from build123d import *

# Parameters (mm, degrees)
BOSS_EXTRUDE1_DEPTH            = 15
CUT_EXTRUDE1_DEPTH             = 5
CBORE_FOR_M3_SHCS1_D           = 3.4
CBORE_FOR_M3_SHCS1_CBORE_D     = 6.5
CBORE_FOR_M3_SHCS1_CBORE_DEPTH = 3
CRVPATTERN1_START              = -15
CRVPATTERN1_OUTLINE_R          = 1.7
CRVPATTERN1_DEPTH              = 30
CRVPATTERN1_START_2            = 12
CRVPATTERN1_2_OUTLINE_R        = 3.25
CRVPATTERN1_2_OUTLINE_R_2      = 1.7
CRVPATTERN1_2_DEPTH            = 3


# Read off the part's stored shape, not the designer's step: CrvPattern1
with BuildPart() as part:
    # Sketch1 → Boss-Extrude1 (new, symmetric)
    with BuildSketch(Plane.XY):
        with BuildLine():
            Line((-100.2, 0), (-100.2, -70))
            Line((-100.2, -70), (-120.2, -70))
            Line((-120.2, -70), (-120.2, 120))
            Line((-120.2, 120), (120.2, 120))
            Line((120.2, 120), (120.2, -70))
            Line((120.2, -70), (100.2, -70))
            Line((100.2, -70), (100.2, 0))
            ThreePointArc((100.2, 0), (0, 100.2), (-100.2, 0))
        make_face()
    extrude(amount=BOSS_EXTRUDE1_DEPTH, both=True)

    # Sketch2 → Cut-Extrude1 (cut, symmetric)
    with BuildSketch(Plane.XY):
        with BuildLine():
            Line((-110.2, -70), (-110.2, 0))
            ThreePointArc((-110.2, 0), (0, 110.2), (110.2, 0))
            Line((110.2, 0), (110.2, -70))
            Line((110.2, -70), (100.2, -70))
            Line((100.2, -70), (100.2, 0))
            ThreePointArc((100.2, 0), (0, 100.2), (-100.2, 0))
            Line((-100.2, 0), (-100.2, -70))
            Line((-100.2, -70), (-110.2, -70))
        make_face()
    extrude(amount=CUT_EXTRUDE1_DEPTH, both=True, mode=Mode.SUBTRACT)

    # CBORE for M3 SHCS1 (through all)
    with Locations(Plane.XY.offset(15)):
        with Locations((-105.2, -55)):
            CounterBoreHole(CBORE_FOR_M3_SHCS1_D / 2, CBORE_FOR_M3_SHCS1_CBORE_D / 2, CBORE_FOR_M3_SHCS1_CBORE_DEPTH)

    # CrvPattern1 outline → CrvPattern1 (cut)
    with BuildSketch(Plane.XY.offset(CRVPATTERN1_START)):
        with Locations((-103.59220022, 18.322010084)):
            Circle(CRVPATTERN1_OUTLINE_R)
        with Locations((-67.600164716, 80.605568855)):
            Circle(CRVPATTERN1_OUTLINE_R)
        with Locations((0, 105.2)):
            Circle(CRVPATTERN1_OUTLINE_R)
        with Locations((67.600164716, 80.605568855)):
            Circle(CRVPATTERN1_OUTLINE_R)
        with Locations((103.59220022, 18.322010084)):
            Circle(CRVPATTERN1_OUTLINE_R)
        with Locations((105.2, -55)):
            Circle(CRVPATTERN1_OUTLINE_R)
    extrude(amount=CRVPATTERN1_DEPTH, mode=Mode.SUBTRACT)

    # CrvPattern1 2 outline → CrvPattern1 2 (cut)
    # profile 1 of 6: a face of its own
    with BuildSketch(Plane.XY.offset(CRVPATTERN1_START_2)):
        with Locations((-103.59220022, 18.322010084)):
            Circle(CRVPATTERN1_2_OUTLINE_R)
        with Locations((-103.59220022, 18.322010084)):
            Circle(CRVPATTERN1_2_OUTLINE_R_2, mode=Mode.SUBTRACT)
    # profile 2 of 6: a face of its own
    with BuildSketch(Plane.XY.offset(CRVPATTERN1_START_2)):
        with Locations((-67.600164716, 80.605568855)):
            Circle(CRVPATTERN1_2_OUTLINE_R)
        with Locations((-67.600164716, 80.605568855)):
            Circle(CRVPATTERN1_2_OUTLINE_R_2, mode=Mode.SUBTRACT)
    # profile 3 of 6: a face of its own
    with BuildSketch(Plane.XY.offset(CRVPATTERN1_START_2)):
        with Locations((0, 105.2)):
            Circle(CRVPATTERN1_2_OUTLINE_R)
        with Locations((0, 105.2)):
            Circle(CRVPATTERN1_2_OUTLINE_R_2, mode=Mode.SUBTRACT)
    # profile 4 of 6: a face of its own
    with BuildSketch(Plane.XY.offset(CRVPATTERN1_START_2)):
        with Locations((67.600164716, 80.605568855)):
            Circle(CRVPATTERN1_2_OUTLINE_R)
        with Locations((67.600164716, 80.605568855)):
            Circle(CRVPATTERN1_2_OUTLINE_R_2, mode=Mode.SUBTRACT)
    # profile 5 of 6: a face of its own
    with BuildSketch(Plane.XY.offset(CRVPATTERN1_START_2)):
        with Locations((103.59220022, 18.322010084)):
            Circle(CRVPATTERN1_2_OUTLINE_R)
        with Locations((103.59220022, 18.322010084)):
            Circle(CRVPATTERN1_2_OUTLINE_R_2, mode=Mode.SUBTRACT)
    # profile 6 of 6: a face of its own
    with BuildSketch(Plane.XY.offset(CRVPATTERN1_START_2)):
        with Locations((105.2, -55)):
            Circle(CRVPATTERN1_2_OUTLINE_R)
        with Locations((105.2, -55)):
            Circle(CRVPATTERN1_2_OUTLINE_R_2, mode=Mode.SUBTRACT)
    extrude(amount=CRVPATTERN1_2_DEPTH, mode=Mode.SUBTRACT)


solid = part.part
Geometry check sheet. Reference: the model listing, model coordinates, mm. A direction names the side the tool comes from. Give positions to 0.01 mm unless a question says otherwise; leave off trailing zeros. Loops run counter-clockwise (first coordinate to the right, second up) from the corner with the lowest first, then second, coordinate; pieces in that order, holes last. Notation, with made-up numbers: (10.5, 86.25) -> (20.5, 86.25) arc R27 cw to (20.5, 107.25) -> close; hole circle Ø8 at (52, -17). An arc over 180 degrees is marked (long way). Answer in a Markdown table with one row per item. Add a question column.
1) Cross-section at B-B on z = 0.25. Record the boundary of the cut face in (x, y).
2) Set-up check for faces 4 (the face through (100.2, -35, 10)), 5 (the face through (1, 101, 5)), 6 (the face through (67.18, 83.83, 13.48)), 7 (the face through (113, -70, 0)): record each of +Z, -Z, +X, -X, +Y, -Y from which the full face is reachable in a straight line by a thin tool's end or side.
3) Gauge pin test, flat ends, axial feed: P1, Ø3, axis at x = 68, y = 81.5, coming from the +Z side; P2, Ø10, axis at x = 75.5, z = -3, coming from the -Y side. Record the tip position at first contact, or that the pin passes through.
4) Material ranges on probe 1 along Z at (x, y) = (-102.5, -56.5); probe 2 along X at (y, z) = (75.5, -6.75); probe 3 along X at (y, z) = (-30, 4.75), recorded low to high. Write a range as from..to.
5) Cross-section at C-C on x = -51. Record the boundary of the cut face in (y, z).
6) Draft check along Z on faces 1 (the face through (108.3, -54.02, 13.48)), 2 (the face through (1, 101, -5)), 3 (the face through (2, 111, 15)). Enter one of: pulls with the +Z half, pulls with the -Z half, needs draft (parallel to the pull), parting line crosses it, or undercut.
7) Cross-section at A-A on y = 56. Record the boundary of the cut face in (x, z).
Outcome:
| question | item | result |
|---|---|---|
| 1 | outline | (-120.2, -70) -> (-110.2, -70) -> (-110.2, 0) arc R110.2 cw to (110.2, 0) -> (110.2, -70) -> (120.2, -70) -> (120.2, 120) -> (-120.2, 120) -> close |
| 2 | face 4 | +Z, -Z, -Y |
| 2 | face 5 | -Y |
| 2 | face 6 | +Z |
| 2 | face 7 | +Z, -Z, +X, -X, -Y |
| 3 | P1 | stops at z = 12 |
| 3 | P2 | stops at y = 60.22 |
| 4 | probe 1 | z = -15..-5, 5..12 |
| 4 | probe 2 | x = -120.2..-65.88, 65.88..120.2 |
| 4 | probe 3 | x = -120.2..-110.2, 110.2..120.2 |
| 5 | outline | (86.25, -15) -> (120, -15) -> (120, 15) -> (86.25, 15) -> (86.25, 5) -> (97.69, 5) -> (97.69, -5) -> (86.25, -5) -> close |
| 6 | face 1 | needs draft |
| 6 | face 2 | undercut |
| 6 | face 3 | pulls with the +Z half |
| 7 | outline | (-120.2, -15) -> (-83.09, -15) -> (-83.09, -5) -> (-94.91, -5) -> (-94.91, 5) -> (-83.09, 5) -> (-83.09, 15) -> (-120.2, 15) -> close; (83.09, -15) -> (120.2, -15) -> (120.2, 15) -> (83.09, 15) -> (83.09, 5) -> (94.91, 5) -> (94.91, -5) -> (83.09, -5) -> close |
